The model under review builds one solid part; all positions refer to its coordinate system, in mm. Face numbers are marked on the shaded views. Round coordinates to 2 decimals unless told otherwise and drop trailing zeros. Order: outer loops, then holes, each group sorted by start corner. A loop starts at its lowest first (then second) coordinate and runs counter-clockwise, first axis right, second up. Notation, with made-up numbers: (52.5, 56.25) -> (57.5, 56.25) arc R28 ccw to (57.5, 86.25) -> close; hole circle Ø7 at (8, -16). An arc over 180 degrees is marked (long way). Put each result on its own line as item: value. Start each with the question number.
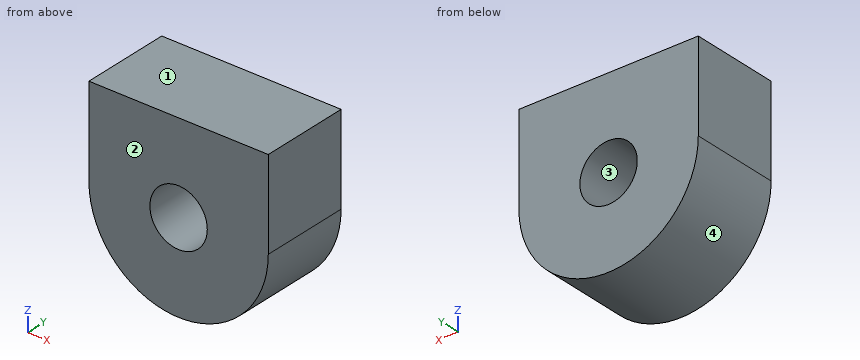
from build123d import *

# Parameters (mm, degrees)
SKETCH1_R           = 3.2
BOSS_EXTRUDE1_DEPTH = 10


with BuildPart() as part:
    # Sketch1 → Boss-Extrude1 (new body)
    with BuildSketch(Plane(origin=(0, 0, 0), x_dir=(1, 0, 0), z_dir=(0, 1, 0))):
        with BuildLine():
            Line((0, 0), (0, -10))
            Line((0, -10), (20, -10))
            Line((20, -10), (20, 0))
            ThreePointArc((20, 0), (10, 10), (0, 0))
        make_face()
        with Locations((10, 0)):
            Circle(SKETCH1_R, mode=Mode.SUBTRACT)
    extrude(amount=-BOSS_EXTRUDE1_DEPTH)


solid = part.part
Q1. Take a section at B-B on y = -9.5. Give the boundary of the cut face in (x, z), and give its area (3 significant figures).
Q2. Take a section at A-A on x = 10. Give the boundary of the cut face in (y, z).
Q3. Clearance check with flat-ended pins moving along their axes: pin 1 Ø2 at (x, z) = (5.5, -3) entering from +Y; pin 2 Ø2 at (x, y) = (12, -6) entering from -Z; pin 3 Ø4 at (x, y) = (3.5, -3) entering from -Z. State where each tip first meets the part, or that it passes through.
Q4. Wall thickness on probe 1 along Z at (x, y) = (10, -4.5); probe 2 along X at (y, z) = (-1.25, 1.75); probe 3 along Z at (x, y) = (9.25, -0.75): over which ranges is each line inside the solid? List them lowest first. Write a range as [from, to].
Q5. Take a section at D-D on z = -4.5. Give the boundary of the cut face in (x, y), and give its area (3 significant figures).
Q6. Draft analysis for pull direction Z (two halves, no side actions). For the marked faces 1, 2, 3 and 4, state which applies: +Z half, -Z half, draft (parallel to the pull), parting line (faces both ways), or undercut.
Q7. Take a section at C-C on x = 12.25. Give the boundary of the cut face in (y, z).
Calculated:
1. outline: (0, 0) arc R10 ccw to (20, 0) -> (20, 10) -> (0, 10) -> close; hole circle Ø6.4 at (10, 0)
1. area: 325 mm²
2. outline: (-10, -10) -> (0, -10) -> (0, -3.2) -> (-10, -3.2) -> close; (-10, 3.2) -> (0, 3.2) -> (0, 10) -> (-10, 10) -> close
3. pin 1: stops at y = 0
3. pin 2: stops at z = -9.95
3. pin 3: stops at z = -8.93
4. probe 1: z = [-10, -3.2], [3.2, 10]
4. probe 2: x = [0, 7.32], [12.68, 20]
4. probe 3: z = [-9.97, -3.11], [3.11, 10]
5. outline: (1.07, -10) -> (18.93, -10) -> (18.93, 0) -> (1.07, 0) -> close
5. area: 179 mm²
6. face 1: +Z half
6. face 2: draft
6. face 3: undercut
6. face 4: -Z half
7. outline: (-10, -9.74) -> (0, -9.74) -> (0, -2.28) -> (-10, -2.28) -> close; (-10, 2.28) -> (0, 2.28) -> (0, 10) -> (-10, 10) -> close
